from build123d import *

# Parameters (mm, degrees)
F1_DEPTH = 3.175
F2_R     = 1.5875
F3_DEPTH = 3.175


with BuildPart() as f1:
    # F0 (on Front) → F1 (new body)
    with BuildSketch(Plane.XZ):
        with BuildLine():
            Line((0, 12.7), (4.576113, 11.846906))
            ThreePointArc((4.576113, 11.846906), (2.327476, 12.484905), (0, 12.7))
        make_face()
        with BuildLine():
            Line((51.381869, 3.121226), (4.576113, 11.846906))
            Line((4.576113, 11.846906), (0, 12.7))
            ThreePointArc((0, 12.7), (-12.7, 0), (0, -12.7))
            Line((0, -12.7), (4.576113, -11.846906))
            Line((4.576113, -11.846906), (51.381869, -3.121226))
            ThreePointArc((51.381869, -3.121226), (53.975, 0), (51.381869, 3.121226))
        make_face()
        with BuildLine():
            Line((4.576113, -11.846906), (0, -12.7))
            ThreePointArc((0, -12.7), (2.327476, -12.484905), (4.576113, -11.846906))
        make_face()
    extrude(amount=F1_DEPTH)

    # F2 (on face) → F3 (join)
    with BuildSketch(Plane.XZ.offset(3.175)):
        with Locations((51.342945, 0)):
            Circle(F2_R)
    extrude(amount=F3_DEPTH)


solid = f1.part
CAD build for the part. Positions are in the model's coordinates, mm. A direction names the side the tool comes from. Round coordinates to 2 decimals unless told otherwise and drop trailing zeros. Write each loop counter-clockwise with the first axis right and the second up, starting at its lowest first coordinate (ties: lowest second). Pieces come first, ordered by that corner, then holes. Notation, with made-up numbers: (-19, -20) -> (15, -20) arc R23 cw to (15, 6) -> close; hole circle Ø2 at (49, -31). An arc over 180 degrees is marked (long way). Answer as a JSON object with one key per item and string values.
(1) Band-saw the part on C-C, the plane x = 21. List the corners of the cut face in (y, z) (3 decimals).
Reported:
{"outline": "(-3.175, -8.785) -> (0, -8.785) -> (0, 8.785) -> (-3.175, 8.785) -> close"}
(2) Pin check, flat tips, straight feed: P1, Ø12, axis at x = 15.5, z = 4.5, coming from the -Y side (3 decimals); P2, Ø4, axis at x = 27, z = -10, coming from the -Y side. Stop position of each tip, or through.
Reported:
{"P1": "stops at y = -3.175", "P2": "passes through"}
(3) Band-saw the part on D-D, the plane z = -6. List the corners of the cut face in (x, y) (3 decimals).
Reported:
{"outline": "(-11.193, -3.175) -> (35.94, -3.175) -> (35.94, 0) -> (-11.193, 0) -> close"}
(4) Which spindle directions (+Z, -Z, +X, -X, +Y, -Y) get a long thin tool onto all of the face, cutting with end or side? Do faces 1 (the face through (53.974, -1.565, -0.062)), 2 (the face through (49.757, -4.74, 0.07)). Say none if no direction does.
Reported:
{"face 1": "+X, +Y, -Y", "face 2": "-Y"}
(5) Band-saw the part on A-A, the plane z = 0. List the corners of the cut face in (x, y) (3 decimals), then the cut area to 3 significant figures.
Reported:
{"outline": "(-12.7, -3.175) -> (49.755, -3.175) -> (49.755, -6.35) -> (52.93, -6.35) -> (52.93, -3.175) -> (53.975, -3.175) -> (53.975, 0) -> (-12.7, 0) -> close", "area": "222 mm^2"}
(6) Probe probe 1 along Z at (x, y) = (-0.5, -0.75); probe 2 along Y at (x, z) = (16.5, -5.5) (3 decimals); probe 3 along Z at (x, y) = (5.5, -0.5). List the from-to ranges inside material, lowest first. Write a range as [from, to].
Reported:
{"probe 1": "z = [-12.69, 12.69]", "probe 2": "y = [-3.175, 0]", "probe 3": "z = [-11.67, 11.67]"}
(7) Band-saw the part on B-B, the plane y = -4.5. List the corners of the cut face in (x, z) (1 decimal).
Reported:
{"outline": "circle Ø3.2 at (51.3, 0)"}
